For this review, take the finished solid that the model builds, in its own axes (mm). A direction names the side the tool comes from. Coordinates: 2 decimals unless noted, no trailing zeros. Write each loop counter-clockwise with the first axis right and the second up, starting at its lowest first coordinate (ties: lowest second). Pieces come first, ordered by that corner, then holes.
```python
from build123d import *

# Parameters (mm, degrees)
PAD006_DEPTH = 10
PAD007_DEPTH = 10


with BuildPart() as clone_of_m3boltslider003:
    # Sketch009 → Pad006 (new body)
    with BuildSketch(Plane.XY):
        with BuildLine():
            ThreePointArc((-1.5, 1.7), (-3.2, 0), (-1.5, -1.7))
            Line((-1.5, -1.7), (1.5, -1.7))
            ThreePointArc((1.5, -1.7), (3.2, 0), (1.5, 1.7))
            Line((-1.5, 1.7), (1.5, 1.7))
        make_face()
    extrude(amount=PAD006_DEPTH)


with BuildPart() as obj1:
    # Sketch010 → Pad007 (new body)
    with BuildSketch(Plane.XY.offset(10)):
        with BuildLine():
            ThreePointArc((-1.5, 2.95), (-4.45, 0), (-1.5, -2.95))
            Line((-1.5, -2.95), (1.5, -2.95))
            ThreePointArc((1.5, -2.95), (4.45, 0), (1.5, 2.95))
            Line((-1.5, 2.95), (1.5, 2.95))
        make_face()
    extrude(amount=PAD007_DEPTH)

    # Fusion015: union Clone of M3BoltSlider003
    add(clone_of_m3boltslider003.part)


solid = obj1.part
```
1) Consider section C-C (z = 9). Give the boundary of the cut face in (x, y).
2) For L1, parallel to Z at x = -2.5, y = 1.5; L2, parallel to Y at x = 1.5, z = 4; L3, parallel to X at y = -1.1, z = 1.25, list the stretches that pass through material, from the lowest coordinate up.
3) Consider section A-A (y = 0). Give the boundary of the cut face in (x, z), then the cut area to 3 significant figures.
4) Consider section B-B (x = 0.75). Give the boundary of the cut face in (y, z), then the cut area to 3 significant figures.
5) Tool access review of faces 1 (the face through (-3.2, 0, 4.9)), 2 (the face through (3.2, 0, 4.9)), 3 (the face through (0, -2, 10)), 4 (the face through (0, 1.7, 5)): name each direction out of +Z, -Z, +X, -X, +Y, -Y from which nothing blocks a thin tool from reaching the whole face with its end or side.
6) Clearance check with flat-ended pins moving along their axes: P1, Ø3.5, axis at x = 0, z = 7, coming from the -Y side; P2, Ø1, axis at y = -1.5, z = 11.5, coming from the -X side; P3, Ø1, axis at x = 1.5, z = 8, coming from the +Y side. State where each tip first meets the part, or that it passes through.
7) Consider section D-D (y = -2.35). Give the boundary of the cut face in (x, z), then the cut area to 3 significant figures.
Results:
1. outline: (-1.5, -1.7) - (1.5, -1.7) arc R1.7 ccw to (1.5, 1.7) - (-1.5, 1.7) arc R1.7 ccw to start
2. L1: z = 10 to 20
2. L2: y = -1.7 to 1.7
2. L3: x = -2.8 to 2.8
3. outline: (-4.45, 10) - (-3.2, 10) - (-3.2, 0) - (3.2, 0) - (3.2, 10) - (4.45, 10) - (4.45, 20) - (-4.45, 20) - close
3. area: 153 mm2
4. outline: (-2.95, 10) - (-1.7, 10) - (-1.7, 0) - (1.7, 0) - (1.7, 10) - (2.95, 10) - (2.95, 20) - (-2.95, 20) - close
4. area: 93.0 mm2
5. face 1: -Z, -X
5. face 2: -Z, +X
5. face 3: -Z
5. face 4: -Z, +X, -X, +Y
6. P1: stops at y = -1.7
6. P2: stops at x = -4.28
6. P3: stops at y = 1.7
7. outline: (-3.28, 10) - (3.28, 10) - (3.28, 20) - (-3.28, 20) - close
7. area: 65.7 mm2
